from build123d import *

# Parameters (mm, degrees)
SKIZZE1_R                       = 10
AUFSATZ_LINEAR_AUSTRAGEN1_DEPTH = 100
SKIZZE2_R                       = 10
SKIZZE2_R_2                     = 8
SCHNITT_LINEAR_AUSTRAGEN1_DEPTH = 68
FASE1_SIZE                      = 2
SKIZZE3_R                       = 10
SKIZZE3_R_2                     = 7.5
SCHNITT_LINEAR_AUSTRAGEN2_DEPTH = 42


with BuildPart() as part:
    # Skizze1 → Aufsatz-Linear austragen1 (new body)
    with BuildSketch(Plane.XY):
        Circle(SKIZZE1_R)
    extrude(amount=AUFSATZ_LINEAR_AUSTRAGEN1_DEPTH)

    # Skizze2 → Schnitt-Linear austragen1 (cut)
    with BuildSketch(Plane.XY.offset(100)):
        Circle(SKIZZE2_R)
        Circle(SKIZZE2_R_2, mode=Mode.SUBTRACT)
    extrude(amount=-SCHNITT_LINEAR_AUSTRAGEN1_DEPTH, mode=Mode.SUBTRACT)

    # Fase1
    fase1_edges = [part.edges().sort_by_distance(p)[0] for p in [
        (-8, 0, 100),
    ]]
    chamfer(fase1_edges, length=FASE1_SIZE)

    # Skizze3 → Schnitt-Linear austragen2 (cut)
    with BuildSketch(Plane(origin=(0, 0, 0), x_dir=(-1, 0, 0), z_dir=(0, 0, -1))):
        Circle(SKIZZE3_R)
        Circle(SKIZZE3_R_2, mode=Mode.SUBTRACT)
    extrude(amount=-SCHNITT_LINEAR_AUSTRAGEN2_DEPTH, mode=Mode.SUBTRACT)


solid = part.part
Design review of the part built by this model. Coordinates are the model's own, in mm. A direction names the side the tool comes from. Give positions to 0.01 mm unless a question says otherwise; leave off trailing zeros. Loops run counter-clockwise (first coordinate to the right, second up) from the corner with the lowest first, then second, coordinate; pieces in that order, holes last. Notation, with made-up numbers: (54.25, -26.5) -> (89.25, -26.5) arc R38 cw to (89.25, 12.5) -> close; hole circle Ø3 at (84.25, -13). An arc over 180 degrees is marked (long way). One line per question, with ' | ' between items. Start each with the question number.
(1) We need section A-A (y = 0). State the section outline as (x, z) points, and give its area (3 significant figures).
(2) For line 1 (X direction, y = -0.5, z = 82); line 2 (Y direction, x = -3.5, z = 83); line 3 (X direction, y = -1.75, z = 80), list the stretches that pass through material, from the lowest coordinate up.
(3) For faces 1 (the face through (-5, -6, 42)), 2 (the face through (-1.73, -7.81, 70.39)), list the 3-axis set-ups (+Z, -Z, +X, -X, +Y, -Y) from which the entire face can be reached by the end or side of a thin tool; tool diameter is ignored.
(4) We need section C-C (z = 47). State the section outline as (x, y) points, and give its area (3 significant figures).
(5) Insertion check: P1, Ø4, axis at x = -3, z = 56, coming from the -Y side; P2, Ø1, axis at x = 0, z = 27, coming from the -Y side; P3, Ø1.5, axis at y = 6.5, z = 21.5, coming from the -X side. Each pin has a flat end and moves straight along its axis. Give the tip position at first contact, or say it passes through.
The answers:
1) outline: (-8, 42) -> (-7.5, 42) -> (-7.5, 0) -> (7.5, 0) -> (7.5, 42) -> (8, 42) -> (8, 98) -> (6, 100) -> (-6, 100) -> (-8, 98) -> close | area: 1,550 mm^2
2) line 1: x = -7.98 to 7.98 | line 2: y = -7.19 to 7.19 | line 3: x = -7.81 to 7.81
3) face 1: -Z | face 2: +Z, -Z
4) outline: circle Ø16 at (0, 0) | area: 201 mm^2
5) P1: stops at y = -7.94 | P2: stops at y = -7.5 | P3: stops at x = -4.82
